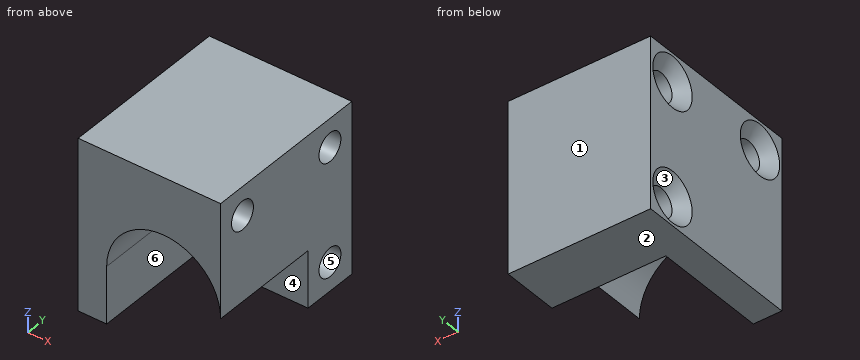
from build123d import *

# Parameters (mm, degrees)
F1_DEPTH = 38.1
F2_DEPTH = 12.7
F3_R     = 3.175
F4_DEPTH = 31.751
F5_SIZE  = 2.54


with BuildPart() as f1:
    # F0 (on Front) → F1 (new body)
    with BuildSketch(Plane.XZ):
        with BuildLine():
            Line((15.875, -6.35), (15.875, 19.05))
            Line((15.875, 19.05), (-15.875, 19.05))
            Line((-15.875, 19.05), (-15.875, -19.05))
            Line((-15.875, -19.05), (-9.525, -19.05))
            Line((-9.525, -19.05), (-9.525, -6.35))
            ThreePointArc((-9.525, -6.35), (3.175, 6.35), (15.875, -6.35))
        make_face()
    extrude(amount=F1_DEPTH)

    # F0 (on Front) → F2 (join)
    with BuildSketch(Plane.XZ):
        with BuildLine():
            ThreePointArc((3.1749999328, -19.05), (12.1552560973, -15.3302561448), (15.875, -6.35))
            ThreePointArc((15.875, -6.35), (3.175, 6.35), (-9.525, -6.35))
            ThreePointArc((-9.525, -6.35), (-5.8052561448, -15.3302560973), (3.1749999328, -19.05))
        make_face()
        with BuildLine():
            Line((15.875, -19.05), (15.875, -6.35))
            ThreePointArc((15.875, -6.35), (12.1552560973, -15.3302561448), (3.1749999328, -19.05))
            Line((3.1749999328, -19.05), (15.875, -19.05))
        make_face()
        with BuildLine():
            ThreePointArc((3.1749999328, -19.05), (-5.8052561448, -15.3302560973), (-9.525, -6.35))
            Line((-9.525, -6.35), (-9.525, -19.05))
            Line((-9.525, -19.05), (3.1749999328, -19.05))
        make_face()
    extrude(amount=F2_DEPTH)

    # F3 (on face) → F4 (cut, through all)
    with BuildSketch(Plane.YZ.offset(15.875)):
        with Locations((-31.75, 12.7)):
            Circle(F3_R)
        with Locations((-6.35, 12.7)):
            Circle(F3_R)
        with Locations((-6.35, -12.7)):
            Circle(F3_R)
    extrude(amount=-F4_DEPTH, mode=Mode.SUBTRACT)

    # F5
    f5_edges = [f1.edges().sort_by_distance(p)[0] for p in [
        (-15.875, -9.525, -12.7),
        (-15.875, -9.525, 12.7),
        (-15.875, -34.925, 12.7),
    ]]
    chamfer(f5_edges, length=F5_SIZE)


solid = f1.part
The listing builds one solid part. Answer for the finished solid, in the listing's coordinates (mm). Face numbers are marked on the shaded views. A direction names the side the tool comes from. Round coordinates to 2 decimals unless told otherwise and drop trailing zeros. Write each loop counter-clockwise with the first axis right and the second up, starting at its lowest first coordinate (ties: lowest second). Pieces come first, ordered by that corner, then holes. Notation, with made-up numbers: M 0,55.25 L 53,55.25 A31 ccw 53,80.25 Z; hole C 30.25,29 d1. An arc over 180 degrees is marked long. Write each question's results on one line, items separated by ' | '. Start each with the question number.
(1) The part is cut by section C-C, the plane x = 11.5. Write down the section's boundary in (y, z) (3 decimals), and give its area (3 significant figures).
(2) Find the intervals of material crossed by line 1 (Z direction, x = 9, y = -5); line 2 (Z direction, x = -13.5, y = -6); line 3 (Y direction, x = -4, z = 11), in increasing order.
(3) The part is cut by section D-D, the plane z = 12.7. Write down the section's boundary in (x, y) (3 decimals), and give its area (3 significant figures).
(4) The part is cut by section A-A, the plane z = -12.7. Write down the section's boundary in (x, y) (3 decimals).
(5) For the marked faces 4, 5 and 6, determine the directions among +Z, -Z, +X, -X, +Y, -Y from which every point of the face is accessible in a straight line to the end or side of a thin tool.
(6) The part is cut by section B-B, the plane y = -6.35. Write down the section's boundary in (x, z) (3 decimals), and give its area (3 significant figures).
(7) Determine the mould class of the marked faces 1, 2 and 3 for opening direction Z: +Z half, -Z half, draft (parallel to the pull), parting line (faces both ways), or undercut.
(8) Each of these flat-tipped pins is pushed along its axis until it touches: P1, Ø5, axis at y = -6.35, z = -12.7, coming from the -X side; P2, Ø2, axis at x = 0.5, y = -26, coming from the -Z side; P3, Ø4, axis at y = -22.5, z = -11, coming from the +X side (3 decimals); P4, Ø8.5, axis at y = -6.35, z = 12.7, coming from the +X side (3 decimals). Where does it stop, or does it pass through?
Worked answers:
1) outline: M -38.1,3.241 L -12.7,3.241 L -12.7,-19.05 L 0,-19.05 L 0,19.05 L -38.1,19.05 Z; hole C -31.75,12.7 d6.35; hole C -6.35,-12.7 d6.35; hole C -6.35,12.7 d6.35 | area: 790 mm²
2) line 1: z = -19.05 to -15.57, -9.83 to 9.83, 15.57 to 19.05 | line 2: z = -19.05 to -16.02, -9.38 to 9.38, 16.02 to 19.05 | line 3: y = -38.1 to -34.43, -29.07 to -9.03, -3.67 to 0
3) outline: M -15.875,-38.1 L 15.875,-38.1 L 15.875,-34.925 L -13.335,-34.925 L -15.875,-37.465 Z; M -15.875,-26.035 L -13.335,-28.575 L 15.875,-28.575 L 15.875,-9.525 L -13.335,-9.525 L -15.875,-12.065 Z; M -15.875,-0.635 L -13.335,-3.175 L 15.875,-3.175 L 15.875,0 L -15.875,0 Z | area: 794 mm²
4) outline: M -15.875,-38.1 L -9.525,-38.1 L -9.525,-12.7 L 15.875,-12.7 L 15.875,-9.525 L -13.335,-9.525 L -15.875,-12.065 Z; M -15.875,-0.635 L -13.335,-3.175 L 15.875,-3.175 L 15.875,0 L -15.875,0 Z
5) face 4: -Z, -Y | face 5: +X, -X | face 6: -Z, +X, -Y
6) outline: M -15.875,-19.05 L 15.875,-19.05 L 15.875,-15.875 L -13.335,-15.875 L -15.875,-18.415 Z; M -15.875,-6.985 L -13.335,-9.525 L 15.875,-9.525 L 15.875,9.525 L -13.335,9.525 L -15.875,6.985 Z; M -15.875,18.415 L -13.335,15.875 L 15.875,15.875 L 15.875,19.05 L -15.875,19.05 Z | area: 794 mm²
7) face 1: draft | face 2: -Z half | face 3: undercut
8) P1: passes through | P2: stops at z = 5.81 | P3: stops at x = -9.525 | P4: stops at x = 15.875
